```python
from build123d import *

# Parameters (mm, degrees)
SKETCH1_R                   = 2.5
BOSS_EXTRUDE1_DEPTH         = 6
SKETCH2_R                   = 4
BOSS_EXTRUDE2_DEPTH         = 1
BOSS_EXTRUDE3_DEPTH         = 1.5
SKETCH7_R                   = 2
BOSS_EXTRUDE4_DEPTH         = 8.5
SKETCH8_R                   = 5.5
CUT_EXTRUDE1_DEPTH          = 0.75
SKETCH9_R                   = 1
CUT_EXTRUDE2_DEPTH          = 57.504424606
M3_TAPPED_HOLE2_D           = 2.5
M3_TAPPED_HOLE2_DEPTH       = 7.5
M3_TAPPED_HOLE2_CSINK_D     = 3.05
M3_TAPPED_HOLE2_CSINK_ANGLE = 90
M3_TAPPED_HOLE2_TIP         = 0.751075774


with BuildPart() as part:
    # Sketch1 → Boss-Extrude1 (new body)
    with BuildSketch(Plane(origin=(0, 0, 0), x_dir=(1, 0, 0), z_dir=(0, 1, 0))):
        with Locations(Location((0, 0, 0), (0, 0, 270))):
            Circle(SKETCH1_R)
    extrude(amount=BOSS_EXTRUDE1_DEPTH)

    # Sketch2 → Boss-Extrude2 (add)
    with BuildSketch(Plane.XZ):
        with Locations(Location((0, 0, 0), (0, 0, 270))):
            Circle(SKETCH2_R)
    extrude(amount=BOSS_EXTRUDE2_DEPTH)



with BuildPart() as body_2:
    # Sketch6 → Boss-Extrude3 (new, symmetric)
    with BuildSketch(Plane(origin=(0, -11, 0), x_dir=(-1, 0, 0), z_dir=(0, -1, 0))):
        with BuildLine():
            ThreePointArc((-5.619513954, -42.214742274), (-0.168678351, -46.073450543), (-6.84690974, -46.02381404))
            ThreePointArc((-6.84690974, -46.02381404), (-24.254725766, -19.04192568), (0, 2))
            ThreePointArc((0, 2), (2, 0), (0, -2))
            ThreePointArc((0, -2), (-20.302736473, -19.662943128), (-5.619513954, -42.214742274))
        make_face()
    extrude(amount=BOSS_EXTRUDE3_DEPTH, both=True)


with BuildPart() as part_1:
    add(part.part)

    add(body_2.part)  # Boss-Extrude4 merges body 2
    # Sketch7 → Boss-Extrude4 (add)
    with BuildSketch(Plane.XZ.offset(1)):
        with Locations(Location((0, 0, 0), (0, 0, 270))):
            Circle(SKETCH7_R)
    extrude(amount=BOSS_EXTRUDE4_DEPTH)

    # Sketch8 → Cut-Extrude1 (cut, symmetric)
    with BuildSketch(Plane(origin=(0, -11, 0), x_dir=(1, 0, 0), z_dir=(0, 1, 0))):
        with Locations((3.5, -45)):
            Circle(SKETCH8_R)
    extrude(amount=CUT_EXTRUDE1_DEPTH, both=True, mode=Mode.SUBTRACT)

    # Sketch9 → Cut-Extrude2 (cut, through all)
    with BuildSketch(Plane(origin=(0, -9.5, 0), x_dir=(1, 0, 0), z_dir=(0, 1, 0))):
        with Locations(Location((3.5, -45, 0), (0, 0, 270))):
            Circle(SKETCH9_R)
    extrude(amount=-CUT_EXTRUDE2_DEPTH, mode=Mode.SUBTRACT)

    # M3 Tapped Hole2
    with Locations(Plane.ZX.offset(6)):
        with Locations((0, 0)):
            CounterSinkHole(M3_TAPPED_HOLE2_D / 2, M3_TAPPED_HOLE2_CSINK_D / 2, depth=M3_TAPPED_HOLE2_DEPTH, counter_sink_angle=M3_TAPPED_HOLE2_CSINK_ANGLE)
            with Locations((0, 0, -(M3_TAPPED_HOLE2_DEPTH + M3_TAPPED_HOLE2_TIP / 2))):  # 118° drill point
                Cone(0, M3_TAPPED_HOLE2_D / 2, M3_TAPPED_HOLE2_TIP, mode=Mode.SUBTRACT)


solid = part_1.part
```
Geometry check sheet. Reference: the model listing, model coordinates, mm. A direction names the side the tool comes from. Coordinates: 2 decimals unless noted, no trailing zeros. Order: outer loops, then holes, each group sorted by start corner. A loop starts at its lowest first (then second) coordinate and runs counter-clockwise, first axis right, second up.
Q1. Tool access check on faces 5 (the face through (-2, -7, 0)), 6 (the face through (4.4, -10.25, 44.2)), 7 (the face through (-2, 6, 0)). Record the directions out of +Z, -Z, +X, -X, +Y, -Y that give a thin tool (end or side, any length) a straight path to the whole face; none if there is none.
Reply:
face 5: none
face 6: +Z, -X
face 7: +Z, -Z, +X, -X, +Y
Q2. Draft check along X on faces 1 (the face through (-0.21, -2.12, -0.05)), 2 (the face through (2, 0, -2)), 3 (the face through (-2.44, 2.96, -0.54)), 4 (the face through (8.73, -10.99, 43.3)). Enter one of: released by +X, released by -X, zero draft, split by the parting line, or undercut.
Reply:
face 1: undercut
face 2: zero draft
face 3: split by the parting line
face 4: released by -X
Q3. Sectioned sample at C-C on y = 3. Record the cut outline in (x, z).
Reply:
outline: circle Ø5 at (0, 0); hole circle Ø2.5 at (0, 0)
Q4. Sectioned sample at B-B on z = 43. Record the cut outline in (x, y).
Reply:
outline: (0.63, -12.5) - (13.42, -12.5) - (13.42, -9.5) - (0.63, -9.5) - (0.63, -10.25) - (8.62, -10.25) - (8.62, -11.75) - (0.63, -11.75) - close
Q5. Thickness scan on probe 1 along Y at (x, z) = (18, 39); probe 2 along Y at (x, z) = (-2.75, 1); probe 3 along Z at (x, y) = (0, -9.25). Record the ranges inside material, lowest first.
Reply:
probe 1: y = -12.5 to -9.5
probe 2: y = -1 to 0
probe 3: z = -2 to 2
Q6. Depth check by flat-ended pin: pin 1 Ø3 at (x, z) = (3.5, 45) entering from +Y; pin 2 Ø1.5 at (x, y) = (2, -2.5) entering from +Z; pin 3 Ø12 at (x, z) = (14, 30) entering from -Y. Enter the tip coordinate at first touch or a pass-through.
Reply:
pin 1: stops at y = -9.5
pin 2: stops at z = 1.56
pin 3: stops at y = -12.5
Q7. Sectioned sample at A-A on x = 16. Record the cut outline in (y, z).
Reply:
outline: (-12.5, 3.95) - (-9.5, 3.95) - (-9.5, 9.68) - (-12.5, 9.68) - close; (-12.5, 35.32) - (-9.5, 35.32) - (-9.5, 41.05) - (-12.5, 41.05) - close
Q8. Sectioned sample at D-D on x = 22. Record the cut outline in (y, z), and give its area (3 significant figures).
Reply:
outline: (-12.5, 11.72) - (-9.5, 11.72) - (-9.5, 33.28) - (-12.5, 33.28) - close
area: 64.7 mm2
